CAD build for the part. Positions are in the model's coordinates, mm. Round coordinates to 2 decimals unless told otherwise and drop trailing zeros. Order: outer loops, then holes, each group sorted by start corner. A loop starts at its lowest first (then second) coordinate and runs counter-clockwise, first axis right, second up. Notation, with made-up numbers: M 32,-7.5 L 50,-7.5 A15 ccw 50,4.5 Z; hole C 65,58 d3. An arc over 180 degrees is marked long. Answer as CSV lines item,"result". Start each with the question number.
```python
from build123d import *

# Parameters (mm, degrees)
BOSS_EXTRUDE1_DEPTH = 812.8
SKETCH2_R           = 14.2875
CUT_EXTRUDE1_DEPTH  = 817.469013879


with BuildPart() as part:
    # Sketch1 → Boss-Extrude1 (new body)
    with BuildSketch(Plane.XY):
        Polygon((0, 0), (0, 69.85), (22.225, 69.85), (22.225, 73.025), (-3.175, 73.025), (-3.175, -3.175), (22.225, -3.175), (22.225, 0), align=None)
    extrude(amount=BOSS_EXTRUDE1_DEPTH)

    # Sketch2 → Cut-Extrude1 (cut, through all)
    with BuildSketch(Plane.ZY.offset(3.175)):
        with Locations(Location((406.4, 34.925, 0), (0, 0, 270))):
            Circle(SKETCH2_R)
        with Locations(Location((152.4, 38.1, 0), (0, 0, 270))):
            Circle(SKETCH2_R)
        with Locations(Location((660.4, 38.1, 0), (0, 0, 270))):
            Circle(SKETCH2_R)
    extrude(amount=-CUT_EXTRUDE1_DEPTH, mode=Mode.SUBTRACT)


solid = part.part
```
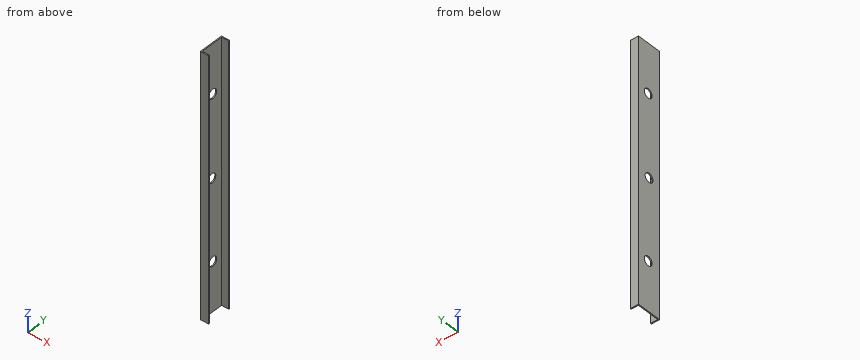
Q1. Probe line 1 along Y through (x, z) = (16.75, 470.5) (3 decimals); line 2 along Z through (x, y) = (-2.3, 38.1); line 3 along Y through (x, z) = (-2.15, 660.4) (1 decimal). List the from-to ranges inside material, lowest first. Write a range as from..to.
Q2. Band-saw the part on B-B, the plane x = 4.25. Write the cut outline in (y, z) (3 decimals), then the cut area to 3 significant figures.
Q3. Band-saw the part on C-C, the plane z = 121.5. Write the cut outline in (x, y) (3 decimals), then the cut area to 3 significant figures.
Q4. Band-saw the part on D-D, the plane y = 38.1. Write the cut outline in (x, z) (1 decimal).
Answer:
1,line 1,"y = -3.175..0, 69.85..73.025"
1,line 2,"z = 0..138.11, 166.69..392.47, 420.33..646.11, 674.69..812.8"
1,line 3,"y = -3.2..23.8, 52.4..73"
2,outline,"M -3.175,0 L 0,0 L 0,812.8 L -3.175,812.8 Z; M 69.85,0 L 73.025,0 L 73.025,812.8 L 69.85,812.8 Z"
2,area,"5,160 mm^2"
3,outline,"M -3.175,-3.175 L 22.225,-3.175 L 22.225,0 L 0,0 L 0,69.85 L 22.225,69.85 L 22.225,73.025 L -3.175,73.025 Z"
3,area,"383 mm^2"
4,outline,"M -3.2,0 L 0,0 L 0,138.1 L -3.2,138.1 Z; M -3.2,166.7 L 0,166.7 L 0,392.5 L -3.2,392.5 Z; M -3.2,420.3 L 0,420.3 L 0,646.1 L -3.2,646.1 Z; M -3.2,674.7 L 0,674.7 L 0,812.8 L -3.2,812.8 Z"
